Read the model definition and answer for the solid it produces. Units are mm, in the model's axes. A direction names the side the tool comes from. Coordinates: 2 decimals unless noted, no trailing zeros. Write each loop counter-clockwise with the first axis right and the second up, starting at its lowest first coordinate (ties: lowest second). Pieces come first, ordered by that corner, then holes.
1) The part is cut by section C-C (z = 224.5). Determine the outline of the cut face in (x, y).
2) Each of these flat-tipped pins is pushed along its axis until it touches: pin 1 Ø3 at (x, z) = (-197, 26) entering from +Y; pin 2 Ø1 at (x, z) = (173.5, -230) entering from -Y. Where does it stop, or does it pass through?
3) The part is cut by section D-D (z = -227). Determine the outline of the cut face in (x, y).
4) The part is cut by section B-B (x = -226.5). Determine the outline of the cut face in (y, z), then the cut area to 3 significant figures.
5) Find the intervals of material crossed by line 1 (X direction, y = 156, z = 254.5); line 2 (X direction, y = -5.5, z = -200); line 3 (Y direction, x = -264, z = -129.5), in increasing order.
6) Which of the six approach directions +Z, -Z, +X, -X, +Y, -Y give full straight-line access (tool end or side, diameter ignored) to faces 1 (the face through (-251, 252, -200)), 2 (the face through (200, 252, -251)), 3 (the face through (-1, 0, -201))?
7) Determine the mould class of faces 4 (the face through (-71, 64, -300)), 5 (the face through (300, 64, 71)), 6 (the face through (-200, 252, 251)) for opening direction X: +X half, -X half, draft (parallel to the pull), parting line (faces both ways), or undercut.
8) The part is cut by section A-A (y = 231.5). Determine the outline of the cut face in (x, z).
from build123d import *

# Parameters (mm, degrees)
SKETCH_1_W          = 600
SKETCH_1_H          = 600
EXTRUDE_1_DEPTH     = 400
CUT_EXTRUDE_1_DEPTH = 300
SKETCH_3_R          = 60
SKETCH_3_R_2        = 50
EXTRUDE_2_DEPTH     = 10


with BuildPart() as part:
    # 草图1 → 凸台-拉伸1 (new body)
    with BuildSketch(Plane(origin=(0, 0, 0), x_dir=(1, 0, 0), z_dir=(0, 1, 0))):
        Rectangle(SKETCH_1_W, SKETCH_1_H)
    extrude(amount=EXTRUDE_1_DEPTH)

    # 草图2 → 切除-拉伸1 (cut)
    with BuildSketch(Plane(origin=(0, 400, 0), x_dir=(1, 0, 0), z_dir=(0, 1, 0))):
        Polygon((-500, 200), (-200, 200), (-200, 500), (200, 500), (200, 200), (500, 200), (500, -200), (200, -200), (200, -500), (-200, -500), (-200, -200), (-500, -200), align=None)
    extrude(amount=-CUT_EXTRUDE_1_DEPTH, mode=Mode.SUBTRACT)

    # 草图3 → 凸台-拉伸2 (add)
    with BuildSketch(Plane.XZ):
        with Locations(Location((0, -200, 0), (0, 0, 90))):
            Circle(SKETCH_3_R)
        with Locations(Location((0, -200, 0), (0, 0, 270))):
            Circle(SKETCH_3_R_2, mode=Mode.SUBTRACT)
    extrude(amount=EXTRUDE_2_DEPTH)


solid = part.part
Reported:
1. outline: (-300, 0) - (300, 0) - (300, 400) - (200, 400) - (200, 100) - (-200, 100) - (-200, 400) - (-300, 400) - close
2. pin 1: stops at y = 100
2. pin 2: stops at y = 0
3. outline: (-300, 0) - (-53.58, 0) - (-53.58, -10) - (-42.08, -10) - (-42.08, 0) - (42.08, 0) - (42.08, -10) - (53.58, -10) - (53.58, 0) - (300, 0) - (300, 400) - (200, 400) - (200, 100) - (-200, 100) - (-200, 400) - (-300, 400) - close
4. outline: (0, -300) - (400, -300) - (400, -200) - (100, -200) - (100, 200) - (400, 200) - (400, 300) - (0, 300) - close
4. area: 120,000 mm2
5. line 1: x = -300 to -200, 200 to 300
5. line 2: x = -60 to -50, 50 to 60
5. line 3: y = 0 to 100
6. face 1: +X, -X, +Y
6. face 2: +Z, -Z, +Y
6. face 3: -Y
7. face 4: draft
7. face 5: +X half
7. face 6: undercut
8. outline: (-300, -300) - (-200, -300) - (-200, -200) - (-300, -200) - close; (-300, 200) - (-200, 200) - (-200, 300) - (-300, 300) - close; (200, -300) - (300, -300) - (300, -200) - (200, -200) - close; (200, 200) - (300, 200) - (300, 300) - (200, 300) - close
